from build123d import *

# Parameters (mm, degrees)
SKETCH1_R           = 10
BOSS_EXTRUDE1_DEPTH = 3
SKETCH2_R           = 5.5
CUT_EXTRUDE1_DEPTH  = 2
SKETCH3_R           = 7
SKETCH4_R           = 3.8
CUT_EXTRUDE2_DEPTH  = 14


with BuildPart() as part:
    # Sketch1 → Boss-Extrude1 (new body)
    with BuildSketch(Plane(origin=(0, 0, 0), x_dir=(0, 0, -1), z_dir=(1, 0, 0))):
        Circle(SKETCH1_R)
    extrude(amount=BOSS_EXTRUDE1_DEPTH)

    # Sketch2 → Cut-Extrude1 (cut)
    with BuildSketch(Plane.ZY):
        Circle(SKETCH2_R)
    extrude(amount=-CUT_EXTRUDE1_DEPTH, mode=Mode.SUBTRACT)

    # Sketch3 → section 0 of loft1
    with BuildSketch(Plane.ZY.offset(-16), mode=Mode.PRIVATE) as loft1_s0:
        Circle(SKETCH3_R)
    # loft up to a face of the part (loft1)
    loft([loft1_s0.sketch, Face(Wire([part.edges().sort_by_distance((3, 7.289686274, 6.845471059))[0]]))])

    # Sketch4 → Cut-Extrude2 (cut)
    with BuildSketch(Plane(origin=(16, 0, 0), x_dir=(0, 0, -1), z_dir=(1, 0, 0))):
        Circle(SKETCH4_R)
    extrude(amount=-CUT_EXTRUDE2_DEPTH, mode=Mode.SUBTRACT)


solid = part.part
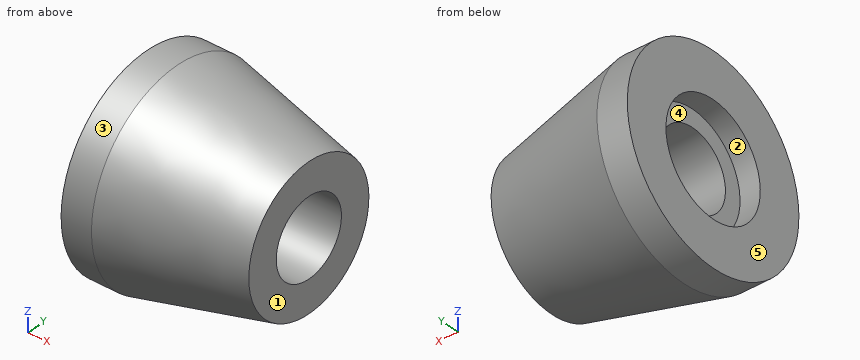
Build history of the part. All positions in model axes, mm. Face numbers are marked on the shaded views. A direction names the side the tool comes from. Give positions to 0.01 mm unless a question says otherwise; leave off trailing zeros. Order: outer loops, then holes, each group sorted by start corner. A loop starts at its lowest first (then second) coordinate and runs counter-clockwise, first axis right, second up. Notation, with made-up numbers: M 46,-8.5 L 91,-8.5 A33 cw 91,23.5 Z; hole C 20,-5 d5. An arc over 180 degrees is marked long. Put each result on its own line as item: value.
Item 1: Probe line 1 (Y direction, x = 0.7, z = 0); line 2 (X direction, y = 4.5, z = 1); line 3 (Y direction, x = 7, z = 1.5). List the from-to ranges inside material, lowest first. Write a range as [from, to].
From the geometry:
line 1: y = [-10, -5.5], [5.5, 10]
line 2: x = [2, 16]
line 3: y = [-8.95, -3.49], [3.49, 8.95]
Item 2: Slice it at A-A, the plane z = 0. Write the cut outline in (x, y), plus the area to 3 significant figures.
From the geometry:
outline: M 0,-10 L 3,-10 L 16,-7 L 16,-3.8 L 2,-3.8 L 2,-5.5 L 0,-5.5 Z; M 0,5.5 L 2,5.5 L 2,3.8 L 16,3.8 L 16,7 L 3,10 L 0,10 Z
area: 153 mm2
Item 3: 3-axis set-ups, long thin cutter, end or side, ignore diameter. For the marked faces 1 and 2: which of +Z, -Z, +X, -X, +Y, -Y reach the whole face in a straight line?
From the geometry:
face 1: +Z, -Z, +X, +Y, -Y
face 2: -X
Item 4: Two-plate mould, pull along Y, no slides. Class the marked faces 3, 4 and 5: +Y half, -Y half, draft (parallel to the pull), parting line (faces both ways), or undercut.
From the geometry:
face 3: parting line
face 4: undercut
face 5: draft
Item 5: Slice it at C-C, the plane x = 15. Write the cut outline in (y, z).
From the geometry:
outline: C 0,0 d14.46; hole C 0,0 d7.6
Item 6: Slice it at B-B, the plane x = 1.5. Write the cut outline in (y, z).
From the geometry:
outline: C 0,0 d20; hole C 0,0 d11
Item 7: Flat gauge pins, fed straight in: pin 1 Ø4 at (x, y) = (3.5, 8) entering from -Z; pin 2 Ø1 at (x, y) = (12, -6) entering from -Z; pin 3 Ø3 at (x, z) = (14, 3.5) entering from +Y; pin 4 Ø3.5 at (y, z) = (0.5, 1) entering from -X. Where does each tip first touch, or does it go through?
From the geometry:
pin 1: stops at z = -7.95
pin 2: stops at z = -5.73
pin 3: stops at y = 7.32
pin 4: passes through
